Geometry: see drawing. Coordinates: mm, zero at the bounding-box minimum. Round coordinates to 2 decimals unless told otherwise and drop trailing zeros. Order: outer loops, then holes, each group sorted by start corner. A loop starts at its lowest first (then second) coordinate and runs counter-clockwise, first axis right, second up. Notation, with made-up numbers: (10.5, 1) - (25.5, 1) arc R16 cw to (25.5, 12) - close; hole circle Ø1 at (43, -35.75). An arc over 180 degrees is marked (long way). Put each result on its own line as item: value. Start each with the question number.
1) Line query: probe 1 along Y at (x, z) = (78, 9.5); probe 2 along Y at (x, z) = (78, 5.75); probe 3 along X at (y, z) = (30, 15.5). Output: solid intervals per line, ascending. Write a range as [from, to].
2) Contact query for flat-ended pins moving along their axis: P1, Ø1.5, axis at y = 10, z = 16, coming from the -X side; P2, Ø10, axis at x = 110, z = 9.5, coming from the -Y side; P3, Ø6, axis at x = 128, z = 11.5, coming from the -Y side; P4, Ø2, axis at x = 103, z = 9, coming from the -Y side. Output: stop coordinate, or through.
3) Section A-A on x = 78. Output: boundary loops of the cut face in (y, z), then the cut area to 3 significant figures.
4) Mould query, pull axis Y, two halves, no side actions, for the marked faces 1, 2 and 3. Classes: +Y half, -Y half, draft (parallel to the pull), parting line (faces both ways), or undercut.
5) Section C-C on z = 9.5. Output: boundary loops of the cut face in (x, y), then the cut area to 3 significant figures.
6) Section B-B on y = 25. Output: boundary loops of the cut face in (x, z), then the cut area to 3 significant figures.
7) Section D-D on x = 136. Output: boundary loops of the cut face in (y, z).
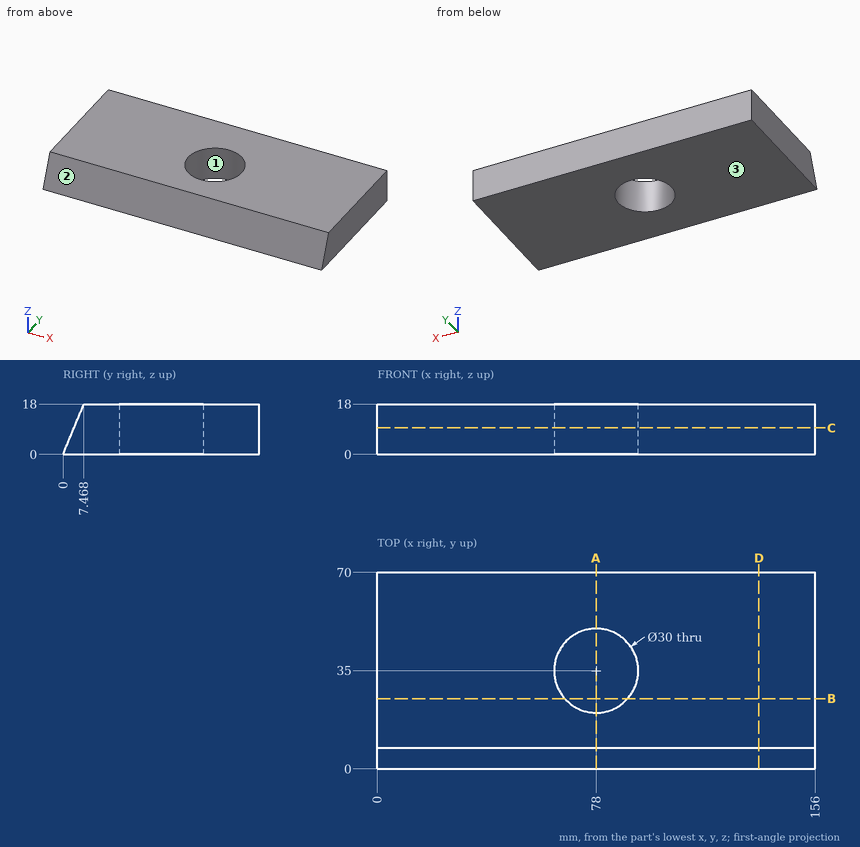
Answer sheet:
1. probe 1: [3.94, 20], [50, 70]
1. probe 2: [2.39, 20], [50, 70]
1. probe 3: [0, 63.86], [92.14, 156]
2. P1: x = 0
2. P2: y = 1.87
2. P3: y = 3.53
2. P4: y = 3.32
3. outline: (0, 0) - (20, 0) - (20, 18) - (7.47, 18) - close; (50, 0) - (70, 0) - (70, 18) - (50, 18) - close
3. area: 653 mm^2
4. face 1: undercut
4. face 2: -Y half
4. face 3: draft
5. outline: (0, 3.94) - (156, 3.94) - (156, 70) - (0, 70) - close; hole circle Ø30 at (78, 35)
5. area: 9,600 mm^2
6. outline: (0, 0) - (66.82, 0) - (66.82, 18) - (0, 18) - close; (89.18, 0) - (156, 0) - (156, 18) - (89.18, 18) - close
6. area: 2,410 mm^2
7. outline: (0, 0) - (70, 0) - (70, 18) - (7.47, 18) - close
